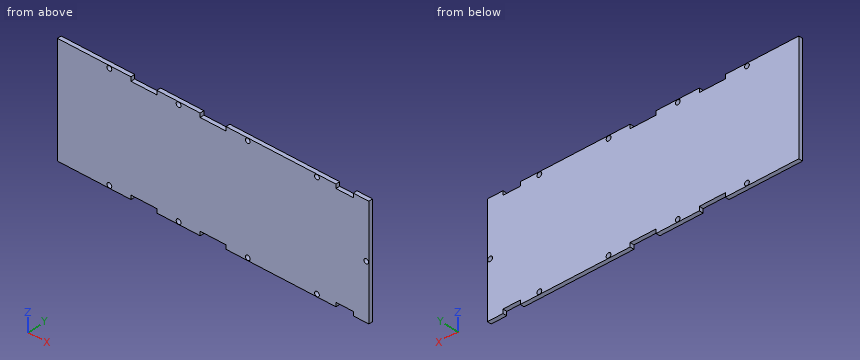
from build123d import *

# Parameters (mm, degrees)
SKETCH1_R           = 1.7526
BOSS_EXTRUDE1_DEPTH = 3


with BuildPart() as part:
    # Sketch1 → Boss-Extrude1 (new body)
    with BuildSketch(Plane(origin=(0, 0, 0), x_dir=(1, 0, 0), z_dir=(0, 1, 0))):
        Polygon((114.3, -0.83215209), (114.3, -41.1), (102.87, -41.1), (102.87, -38.1), (90.17, -38.1), (90.17, -41.1), (89.493211941, -41.1), (77.528882775, -41.1), (74.871117225, -41.1), (26.728882775, -41.1), (24.071117225, -41.1), (9.525, -41.1), (9.525, -38.1), (-9.525, -38.1), (-9.525, -41.1), (-24.071117225, -41.1), (-26.728882775, -41.1), (-41.275, -41.1), (-41.275, -38.1), (-60.325, -38.1), (-60.325, -41.1), (-74.871117225, -41.1), (-77.528882775, -41.1), (-114.3, -41.1), (-114.3, 41.1), (-77.528882775, 41.1), (-74.871117225, 41.1), (-60.325, 41.1), (-60.325, 38.1), (-41.275, 38.1), (-41.275, 41.1), (-26.728882775, 41.1), (-24.071117225, 41.1), (-9.525, 41.1), (-9.525, 38.1), (9.525, 38.1), (9.525, 41.1), (24.071117225, 41.1), (26.728882775, 41.1), (74.871117225, 41.1), (77.528882775, 41.1), (89.493211941, 41.1), (90.17, 41.1), (90.17, 38.1), (102.87, 38.1), (102.87, 41.1), (114.3, 41.1), (114.3, 1.18215209), align=None)
        with Locations((-25.4, -39.195)):
            Circle(SKETCH1_R, mode=Mode.SUBTRACT)
        with Locations((112.395, 0)):
            Circle(SKETCH1_R, mode=Mode.SUBTRACT)
        with Locations((25.4, -39.195)):
            Circle(SKETCH1_R, mode=Mode.SUBTRACT)
        with Locations((76.2, -39.195)):
            Circle(SKETCH1_R, mode=Mode.SUBTRACT)
        with Locations((76.2, 39.195)):
            Circle(SKETCH1_R, mode=Mode.SUBTRACT)
        with Locations((25.4, 39.195)):
            Circle(SKETCH1_R, mode=Mode.SUBTRACT)
        with Locations((-25.4, 39.195)):
            Circle(SKETCH1_R, mode=Mode.SUBTRACT)
        with Locations((-76.2, 39.195)):
            Circle(SKETCH1_R, mode=Mode.SUBTRACT)
        with Locations((-76.2, -39.195)):
            Circle(SKETCH1_R, mode=Mode.SUBTRACT)
    extrude(amount=BOSS_EXTRUDE1_DEPTH)


solid = part.part
CAD build for the part. Positions are in the model's coordinates, mm. Round coordinates to 2 decimals unless told otherwise and drop trailing zeros. Write each loop counter-clockwise with the first axis right and the second up, starting at its lowest first coordinate (ties: lowest second). Pieces come first, ordered by that corner, then holes. Notation, with made-up numbers: M 89,0 L 139,0 A24 cw 139,15 Z; hole C 74.25,46 d1. An arc over 180 degrees is marked long. Put each result on its own line as item: value. Start each with the question number.
1) Drill centre lines: probe 1 along Z at (x, y) = (76.2, 2.3); probe 2 along X at (y, z) = (0.75, 0); probe 3 along Z at (x, y) = (100.5, 1.2). Where is each one in solid material? Low to high. Write a range as [from, to].
2) Saw through at A-A, the plane x = 7. Write the cut outline in (y, z).
3) Pin check, flat tips, straight feed: pin 1 Ø4 at (x, z) = (25.4, 39.195) entering from +Y; pin 2 Ø0.9 at (x, y) = (97, 1) entering from -Z. Stop position of each tip, or through.
4) Saw through at B-B, the plane y = 2.25. Count the separate pieces of the cut face and the enclosed holes in it, and give its area (3 significant figures).
Resolved:
1. probe 1: [-41.1, -40.95], [-37.44, 37.44], [40.95, 41.1]
1. probe 2: [-114.3, 110.64], [114.15, 114.3]
1. probe 3: [-38.1, 38.1]
2. outline: M 0,-38.1 L 3,-38.1 L 3,38.1 L 0,38.1 Z
3. pin 1: y = 3
3. pin 2: z = -38.1
4. separate pieces: 1
4. enclosed holes: 9
4. area: 18,400 mm²
